Could you check a few things on this model? Use its own coordinates, in mm. Face numbers are marked on the shaded views. A direction names the side the tool comes from. Give positions to 0.01 mm unless a question says otherwise; leave off trailing zeros. Loops run counter-clockwise (first coordinate to the right, second up) from the corner with the lowest first, then second, coordinate; pieces in that order, holes last. Notation, with made-up numbers: M -20,-2.75 L -10,-2.75 A20 ccw -10,23.25 Z; hole C -19,30.5 d1. An arc over 180 degrees is marked long. Return JSON: item names as keys, results as strings. Group by question number.
1. If we section it at B-B (z = 17): Write out the boundary of the cut face in (x, y), plus the area to 3 significant figures.
2. For the marked faces 1 and 2, which set-ups out of +Z, -Z, +X, -X, +Y, -Y let a thin tool reach every point of the face, with its end or its side?
3. If we section it at D-D (z = 25): Write out the boundary of the cut face in (x, y), plus the area to 3 significant figures.
4. For pin 1 (0.5 mm diameter, centred on x = -1.5, z = -10, fed in from -Y); pin 2 (2 mm diameter, centred on x = 2.5, y = -85.5, fed in from -Z); pin 3 (8 mm diameter, centred on y = -87, z = -10, fed in from -X), each with a flat end and sliding along its axis, tell me the tip position at first contact or that it passes through.
5. Please list where these lines run through material, in increasing order: line 1 (Y direction, x = -58, z = 1.5); line 2 (Z direction, x = -0.5, y = -32); line 3 (Y direction, x = 30, z = 0).
6. If we section it at A-A (y = -21): Write out the boundary of the cut face in (x, z), plus the area to 3 significant figures.
7. If we section it at C-C (x = -49): Write out the boundary of the cut face in (y, z).
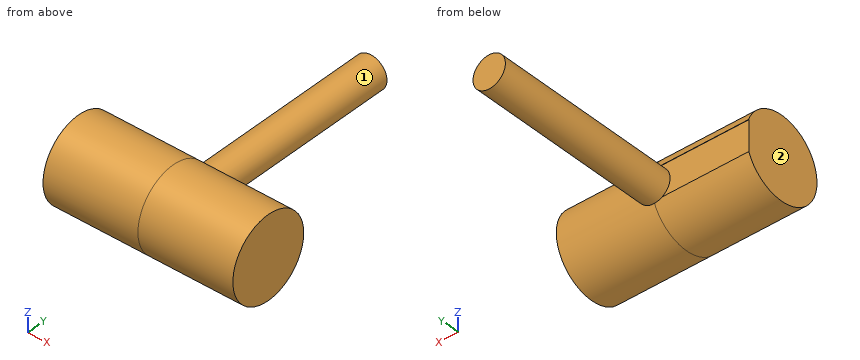
```python
from build123d import *

# Parameters (mm, degrees)
F0_R      = 10.839936
F1_DEPTH  = 50.8
F1_FACE_R = 10.839936
F2_DEPTH  = 76.2
F3_R      = 27.326427
F4_DEPTH  = 63.5
F5_DEPTH  = 63.5


with BuildPart() as f1:
    # F0 (on Front) → F1 (new body)
    with BuildSketch(Plane.XZ):
        Circle(F0_R)
    extrude(amount=F1_DEPTH)

    # F1_face (on face) → F2 (join)
    with BuildSketch(Plane.XZ.offset(50.8)):
        Circle(F1_FACE_R)
    extrude(amount=F2_DEPTH)

    # F3 (on Right) → F4 (join)
    with BuildSketch(Plane.YZ):
        with Locations((-152.289372, 1.042985)):
            Circle(F3_R)
    extrude(amount=F4_DEPTH)

    # F4_face (on face) → F5 (join)
    with BuildSketch(Plane(origin=(0, -152.607876, 1.043252), x_dir=(0, 1, 0), z_dir=(-1, 0, 0))):
        with BuildLine():
            Line((25.828372, -9.796684), (25.607876, -9.796684))
            Line((25.607876, -9.796684), (25.607876, 10.353106))
            ThreePointArc((25.607876, 10.353106), (-27.006288, -0.298744), (25.828372, -9.796684))
        make_face()
    extrude(amount=F5_DEPTH)


solid = f1.part
```
Answer:
{
 "1": {"outline": "M -63.5,-174.47 L 63.5,-174.47 L 63.5,-130.11 L -63.5,-130.11 Z", "area": "5,630 mm²"},
 "2": {"face 1": "+Y", "face 2": "+Z, -Z, -X, +Y, -Y"},
 "3": {"outline": "M -63.5,-165.43 L 63.5,-165.43 L 63.5,-139.14 L -63.5,-139.14 Z", "area": "3,340 mm²"},
 "4": {"pin 1": "stops at y = -177.39", "pin 2": "stops at z = -10.74", "pin 3": "stops at x = -9.03"},
 "5": {"line 1": "y = -179.61 to -127", "line 2": "z = -10.83 to 10.83", "line 3": "y = -179.6 to -124.98"},
 "6": {"outline": "C 0,0 d21.68", "area": "369 mm²"},
 "7": {"outline": "M -127,-9.31 L -127,10.84 L -126.78,10.84 A27.33 ccw long Z"}
}
